from build123d import *

# Parameters (mm, degrees)
CIRPATTERN1_COUNT = 6


with BuildPart() as part:
    # Sketch1 → Revolve1 (revolve)
    with BuildSketch(Plane(origin=(0, 0, 0), x_dir=(0, 0, -1), z_dir=(1, 0, 0)), mode=Mode.PRIVATE) as revolve1_sk:
        with BuildLine():
            Line((-8, 16.4), (-4.594744112, 18.366025404))
            ThreePointArc((-4.594744112, 18.366025404), (-4.353563157, 18.465925826), (-4.094744112, 18.5))
            Line((-4.094744112, 18.5), (9, 18.5))
            Line((9, 18.5), (9, 17.5))
            Line((9, 17.5), (0, 17.5))
            Line((0, 17.5), (0, 11))
            Line((0, 11), (-1.5, 11))
            Line((-1.5, 11), (-1.5, 16.5))
            ThreePointArc((-1.5, 16.5), (-1.792893219, 17.207106781), (-2.5, 17.5))
            Line((-2.5, 17.5), (-3.326794919, 17.5))
            ThreePointArc((-3.326794919, 17.5), (-3.585613964, 17.465925826), (-3.826794919, 17.366025404))
            Line((-3.826794919, 17.366025404), (-5.5, 16.4))
            Line((-5.5, 16.4), (-8, 16.4))
        make_face()
    revolve(revolve1_sk.sketch.rotate(Axis((0, 0, 0), (0, 0, 1)), 90), axis=Axis((0, 0, 0), (0, 0, 1)))

    # Sketch2 → M2.5 Clearance Hole1 (revolve, cut)
    with BuildSketch(Plane(origin=(0, 13, 1.5), x_dir=(0, -1, 0), z_dir=(1, 0, 0))):
        Polygon((0, 0), (0, 23.871247898), (1.45, 23), (1.45, 0), align=None)
    m2_5_clearance_hole1 = revolve(axis=Axis((0, 13, 7.85), (0, 0, -1)), mode=Mode.SUBTRACT)

    # CirPattern1: M2.5 Clearance Hole1 ×6 about axis
    cirpattern1_axis = Axis((0, 0, 0), (0, 0, 1))
    for i in range(1, CIRPATTERN1_COUNT):
        add(m2_5_clearance_hole1.rotate(cirpattern1_axis, i * 360 / CIRPATTERN1_COUNT), mode=Mode.SUBTRACT)


solid = part.part
CAD build for the part. Positions are in the model's coordinates, mm. A direction names the side the tool comes from. Give positions to 0.01 mm unless a question says otherwise; leave off trailing zeros. Loops run counter-clockwise (first coordinate to the right, second up) from the corner with the lowest first, then second, coordinate; pieces in that order, holes last. Notation, with made-up numbers: M 73.25,89 L 131.25,89 A9 cw 131.25,97 Z; hole C -32.75,84 d7. An arc over 180 degrees is marked long. Answer in a Markdown table with one row per item. Add a question column.
Item 1: Band-saw the part on A-A on x = 0. Give the number of separate pieces and of enclosed holes in the cut face, then the cut area to 3 significant figures.
Item 2: Mould opens along X. For faces 1 (the face through (-9.82, 6.31, 0.76)), 2 (the face through (-8.54, 16.41, -2.54)), 3 (the face through (11, 14, -9)) say: +X half, -X half, draft (parallel to the pull), parting line (faces both ways), or undercut.
Item 3: Drop flat-ended pins along their axis: P1, Ø4, axis at x = 0, y = -13, coming from the +Z side; P2, Ø1.5, axis at x = 5, z = -5.5, coming from the +Y side; P3, Ø2, axis at x = -11.5, z = -5.5, coming from the -Y side. Give the stop position or say it passes through.
Item 4: Tool access for faces 4 (the face through (3.794, 17.084, 2.919)), 5 (the face through (2.13, -16.26, 6.77)), 6 (the face through (-9.84, -6.19, 0.76)), 7 (the face through (3.794, 17.084, -4.437)): list every direction of +Z, -Z, +X, -X, +Y, -Y with a clear straight run to the whole face (end or side of a thin tool).
Item 5: Band-saw the part on B-B on z = -5.25. Give the cut face in (x, y).
Item 6: Probe probe 1 along X at (y, z) = (6.5, 0.4); probe 2 along Y at (x, z) = (0, 3.25); probe 3 along Z at (x, y) = (-3.5, 11.5). List the from-to ranges inside material, lowest first.
Reply:
| question | item | result |
|---|---|---|
| 1 | separate pieces | 4 |
| 1 | enclosed holes | 0 |
| 1 | area | 45.2 mm^2 |
| 2 | face 1 | undercut |
| 2 | face 2 | parting line |
| 2 | face 3 | draft |
| 3 | P1 | stops at z = 1.5 |
| 3 | P2 | stops at y = 18.01 |
| 3 | P3 | stops at y = -15.23 |
| 4 | face 4 | none |
| 4 | face 5 | +Z |
| 4 | face 6 | +Z, -Z |
| 4 | face 7 | -Z |
| 5 | outline | C 0,0 d37; hole C 0,0 d35 |
| 6 | probe 1 | x = -17.32 to -12.71, -9.81 to -8.87, 8.87 to 9.81, 12.71 to 17.32 |
| 6 | probe 2 | y = -18.5 to -17.5, 17.5 to 18.5 |
| 6 | probe 3 | z = 0 to 1.5 |
